from build123d import *

# Parameters (mm, degrees)
F0_W            = 25
F0_H            = 20
F1_DEPTH        = 2.5
F3_DEPTH        = 5
F5_DEPTH        = 5
F6_R            = 1.15
F7_DEPTH        = 10
F8_SIZE2        = 2
F8_SIZE         = 3
F10_D           = 3.5
F10_CSINK_D     = 6
F10_CSINK_ANGLE = 90


with BuildPart() as f1:
    # F0 (on Top) → F1 (new body, symmetric)
    with BuildSketch(Plane.XY):
        Rectangle(F0_W, F0_H)
    extrude(amount=F1_DEPTH, both=True)

    # F2 (on face) → F3 (join)
    with BuildSketch(Plane(origin=(0, 10, 0), x_dir=(-1, 0, 0), z_dir=(0, 1, 0))):
        with BuildLine():
            ThreePointArc((15, -2.5), (16.767767, -1.767767), (17.5, 0))
            ThreePointArc((17.5, 0), (16.767767, 1.767767), (15, 2.5))
            ThreePointArc((15, 2.5), (13.232233, 1.767767), (12.5, 0))
            ThreePointArc((12.5, 0), (13.232233, -1.767767), (15, -2.5))
        make_face()
        with BuildLine():
            ThreePointArc((12.5, 0), (13.232233, 1.767767), (15, 2.5))
            Line((15, 2.5), (12.5, 2.5))
            Line((12.5, 2.5), (12.5, 0))
        make_face()
        with BuildLine():
            Line((12.5, -2.5), (15, -2.5))
            ThreePointArc((15, -2.5), (13.232233, -1.767767), (12.5, 0))
            Line((12.5, 0), (12.5, -2.5))
        make_face()
    extrude(amount=-F3_DEPTH)

    # F4 (on face) → F5 (join)
    with BuildSketch(Plane.XZ.offset(10)):
        with BuildLine():
            ThreePointArc((-15, -2.5), (-13.232233, -1.767767), (-12.5, 0))
            ThreePointArc((-12.5, 0), (-13.232233, 1.767767), (-15, 2.5))
            ThreePointArc((-15, 2.5), (-17.5, 0), (-15, -2.5))
        make_face()
        with BuildLine():
            Line((-12.5, -2.5), (-12.5, 0))
            ThreePointArc((-12.5, 0), (-13.232233, -1.767767), (-15, -2.5))
            Line((-15, -2.5), (-12.5, -2.5))
        make_face()
        with BuildLine():
            ThreePointArc((-15, 2.5), (-13.232233, 1.767767), (-12.5, 0))
            Line((-12.5, 0), (-12.5, 2.5))
            Line((-12.5, 2.5), (-15, 2.5))
        make_face()
    extrude(amount=-F5_DEPTH)

    # F6 (on face) → F7 (join)
    with BuildSketch(Plane(origin=(0, -5, 0), x_dir=(-1, 0, 0), z_dir=(0, 1, 0))):
        with Locations((15.2, 0)):
            Circle(F6_R)
    extrude(amount=F7_DEPTH)

    # F8
    f8_edges = [f1.edges().sort_by_distance(p)[0] for p in [
        (-12.5, 0, -2.5),
        (-12.5, 0, 2.5),
    ]]
    chamfer(f8_edges, length=F8_SIZE, length2=F8_SIZE2)

    # F10 (through all)
    with Locations(Plane.XY.offset(2.5)):
        with Locations((-4, 0), (7, 0)):
            CounterSinkHole(F10_D / 2, F10_CSINK_D / 2, counter_sink_angle=F10_CSINK_ANGLE)


solid = f1.part
The listing builds one solid part. Answer for the finished solid, in the listing's coordinates (mm). A direction names the side the tool comes from. Round coordinates to 2 decimals unless told otherwise and drop trailing zeros. Write each loop counter-clockwise with the first axis right and the second up, starting at its lowest first coordinate (ties: lowest second). Pieces come first, ordered by that corner, then holes. Notation, with made-up numbers: (12.25, 5) - (71.25, 5) arc R31 ccw to (71.25, 38) - close; hole circle Ø3 at (45.5, -32). An arc over 180 degrees is marked (long way). Use one line per item in the form item = value. Start each with the question number.
Item 1: A cutting plane is placed at A-A (y = -4.25). Write down the section's boundary in (x, z), plus the area to 3 significant figures.
Item 2: Determine the mould class of faces 1 (the flat face through (-3, -10, 0)), 2 (the flat face through (12.5, 0, 0)), 3 (the flat face through (-13, 5, 0)) for opening direction Y: +Y half, -Y half, draft (parallel to the pull), parting line (faces both ways), or undercut.
Item 3: A cutting plane is placed at D-D (z = -1.85). Write down the section's boundary in (x, y) (3 decimals).
Item 4: A cutting plane is placed at B-B (x = -4). Write down the section's boundary in (y, z).
Item 5: A tool of negligible diameter and unlimited length cuts with its end or side. For faces 4 (the flat face through (-11, -0.1, 1.5)), 5 (the flat face through (-12.5, 0, 0)), 6 (the flat face through (-11, -0.1, -1.5)), 7 (the flat face through (-13.6, -5, 0)), from which of +Z, -Z, +X, -X, +Y, -Y can it reach the whole face along a straight path? Write none if from no direction.
Item 6: Flat-ended cylindrical pins translate along their axes: pin 1 Ø2 at (y, z) = (4.5, 1) entering from -X; pin 2 Ø1.1 at (y, z) = (-0.5, 0) entering from -X. Find the tip coordinate at first contact, or state that the pin passes through.
Item 7: Find the intervals of material crossed by line 1 (Y direction, x = 7, z = -0.9); line 2 (X direction, y = 0, z = -0.65) (3 decimals); line 3 (X direction, y = 0.25, z = 0.85) (3 decimals), in increasing order. Write a range as [from, to].
Item 8: A cutting plane is placed at C-C (y = 0). Write down the section's boundary in (x, z).
The answers:
q1.outline = circle Ø2.3 at (-15.2, 0); (-12.5, -0.5) - (-9.5, -2.5) - (12.5, -2.5) - (12.5, 2.5) - (-9.5, 2.5) - (-12.5, 0.5) - close
q1.area = 123 mm^2
q2.face_1 = -Y half
q2.face_2 = draft
q2.face_3 = undercut
q3.outline = (-16.682, -10) - (12.5, -10) - (12.5, 10) - (-16.682, 10) - (-16.682, 5) - (-10.475, 5) - (-10.475, -5) - (-16.682, -5) - close; hole circle Ø3.5 at (-4, 0); hole circle Ø3.5 at (7, 0)
q4.outline = (-10, -2.5) - (-1.75, -2.5) - (-1.75, 1.25) - (-3, 2.5) - (-10, 2.5) - close; (1.75, -2.5) - (10, -2.5) - (10, 2.5) - (3, 2.5) - (1.75, 1.25) - close
q5.face_4 = +Z
q5.face_5 = +Z, -Z
q5.face_6 = -Z
q5.face_7 = none
q6.pin_1 = -17.5
q6.pin_2 = -16.35
q7.line_1 = [-10, -1.75], [1.75, 10]
q7.line_2 = [-16.149, -14.251], [-12.275, -5.75], [-2.25, 5.25], [8.75, 12.5]
q7.line_3 = [-15.975, -14.425], [-11.975, -5.732], [-2.268, 5.268], [8.732, 12.5]
q8.outline = circle Ø2.3 at (-15.2, 0); (-12.5, -0.5) - (-9.5, -2.5) - (-5.75, -2.5) - (-5.75, 1.25) - (-7, 2.5) - (-9.5, 2.5) - (-12.5, 0.5) - close; (-2.25, -2.5) - (5.25, -2.5) - (5.25, 1.25) - (4, 2.5) - (-1, 2.5) - (-2.25, 1.25) - close; (8.75, -2.5) - (12.5, -2.5) - (12.5, 2.5) - (10, 2.5) - (8.75, 1.25) - close
